```python
from build123d import *

# Parameters (mm, degrees)
F0_W     = 15
F0_H     = 44
F0_W_2   = 9
F0_H_2   = 38
F1_DEPTH = 3.5
F2_R     = 1
F3_R     = 5
F4_R     = 0.5
F5_R     = 1


with BuildPart() as f1:
    # F0 (on Top) → F1 (new body)
    with BuildSketch(Plane.XY):
        Rectangle(F0_W, F0_H)
        Rectangle(F0_W_2, F0_H_2, mode=Mode.SUBTRACT)
    extrude(amount=F1_DEPTH)

    # F2
    f2_edges = [f1.edges().sort_by_distance(p)[0] for p in [
        (4.5, 19, 1.75),
        (-4.5, 19, 1.75),
        (-4.5, -19, 1.75),
        (4.5, -19, 1.75),
    ]]
    fillet(f2_edges, radius=F2_R)

    # F3
    f3_edges = [f1.edges().sort_by_distance(p)[0] for p in [
        (-7.5, -22, 1.75),
        (7.5, -22, 1.75),
        (-7.5, 22, 1.75),
        (7.5, 22, 1.75),
    ]]
    fillet(f3_edges, radius=F3_R)

    # F4
    f4_edges = [f1.edges().sort_by_distance(p)[0] for p in [
        (0, 19, 0),
        (0, 19, 3.5),
    ]]
    fillet(f4_edges, radius=F4_R)

    # F5
    f5_edges = [f1.edges().sort_by_distance(p)[0] for p in [
        (0, -22, 3.5),
        (0, -22, 0),
    ]]
    fillet(f5_edges, radius=F5_R)


solid = f1.part
```
Could you check a few things on this model? Use its own coordinates, in mm. A direction names the side the tool comes from. Round coordinates to 2 decimals unless told otherwise and drop trailing zeros. Loops run counter-clockwise (first coordinate to the right, second up) from the corner with the lowest first, then second, coordinate; pieces in that order, holes last. Notation, with made-up numbers: (85.5, -25.75) - (101.5, -25.75) arc R28 cw to (101.5, 13.25) - close; hole circle Ø9 at (6, 44). An arc over 180 degrees is marked (long way). Use CSV: the item, a comma, the result in double quotes.
Item 1: If we mould it in two halves opening along Y, with no side actions, what happens to faces 3 (the flat face through (0, 22, 2)), 4 (the cylindrical face through (-6.07, -20.5, 1.76)), 5 (the cylindrical face through (4.215, 18.699, 1.767))? For each: pulls with the +Y half, pulls with the -Y half, needs draft (parallel to the pull), parting line crosses it, or undercut.
Here are the results:
face 3,"pulls with the +Y half"
face 4,"pulls with the -Y half"
face 5,"undercut"
Item 2: If we section it at C-C on x = 1: List the corners of the cut face in (y, z) for me, then the cut area to 3 significant figures.
Here are the results:
outline,"(-22, 1) arc R1 ccw to (-21, 0) - (-19.5, 0) arc R0.5 ccw to (-19, 0.5) - (-19, 3) arc R0.5 ccw to (-19.5, 3.5) - (-21, 3.5) arc R1 ccw to (-22, 2.5) - close; (19, 0.5) arc R0.5 ccw to (19.5, 0) - (21, 0) arc R1 ccw to (22, 1) - (22, 2.5) arc R1 ccw to (21, 3.5) - (19.5, 3.5) arc R0.5 ccw to (19, 3) - close"
area,"19.9 mm²"
Item 3: For faces 1 (the flat face through (-4.5, 0, 2)), 2 (the cylindrical face through (6, -20.57, 1.76)), which set-ups out of +Z, -Z, +X, -X, +Y, -Y let a thin tool reach every point of the face, with its end or its side?
Here are the results:
face 1,"+Z, -Z"
face 2,"+Z, -Z, +X, -Y"
Item 4: I need wall thicknesses on L1, parallel to Y at x = -2, z = 2.4; L2, parallel to X at y = 6, z = 1.9; L3, parallel to Y at x = 3.5, z = 2.5. Which ranges of each line are inside material? Lowest first, please. Write a range as [from, to].
Here are the results:
L1,"y = [-22, -19], [19, 22]"
L2,"x = [-7.5, -4.5], [4.5, 7.5]"
L3,"y = [-21.9, -19], [19, 21.9]"
Item 5: If we section it at A-A on z = 1.8: List the corners of the cut face in (x, y) for me, then the cut area to 3 significant figures.
Here are the results:
outline,"(-7.5, -17) arc R5 ccw to (-2.5, -22) - (2.5, -22) arc R5 ccw to (7.5, -17) - (7.5, 17) arc R5 ccw to (2.5, 22) - (-2.5, 22) arc R5 ccw to (-7.5, 17) - close; hole (-4.5, -18) arc R1 ccw to (-3.5, -19) - (3.5, -19) arc R1 ccw to (4.5, -18) - (4.5, 18) arc R1 ccw to (3.5, 19) - (-3.5, 19) arc R1 ccw to (-4.5, 18) - close"
area,"297 mm²"
Item 6: Will this pin go through, and if not, where does the flat tip stop? pin 1 (1 mm diameter, centred on x = 4.5, z = 2, fed in from -Y).
Here are the results:
pin 1,"stops at y = -21.77"
Item 7: If we section it at B-B on y = 9: List the corners of the cut face in (x, z) for me.
Here are the results:
outline,"(-7.5, 1) arc R1 ccw to (-6.5, 0) - (-5, 0) arc R0.5 ccw to (-4.5, 0.5) - (-4.5, 3) arc R0.5 ccw to (-5, 3.5) - (-6.5, 3.5) arc R1 ccw to (-7.5, 2.5) - close; (4.5, 0.5) arc R0.5 ccw to (5, 0) - (6.5, 0) arc R1 ccw to (7.5, 1) - (7.5, 2.5) arc R1 ccw to (6.5, 3.5) - (5, 3.5) arc R0.5 ccw to (4.5, 3) - close"
